Verification items for the finished model (mm, model axes). Give positions to 0.01 mm unless a question says otherwise; leave off trailing zeros. Order: outer loops, then holes, each group sorted by start corner. A loop starts at its lowest first (then second) coordinate and runs counter-clockwise, first axis right, second up. Notation, with made-up numbers: (27, 62.5) -> (48, 62.5) arc R10 cw to (48, 68.5) -> close; hole circle Ø6 at (51.25, 2.5). An arc over 180 degrees is marked (long way). Return JSON: item names as keys, results as strings. Group by question number.
(1) Cross-section at A-A on y = 1.75. Enter the section's corners in (x, z).
(2) Cross-section at B-B on x = 0. State how many separate pieces and enclosed holes the cut face has, then the cut area to 3 significant figures.
(3) Thickness scan on line 1 along Z through (x, y) = (0, 4.45); line 2 along X through (y, z) = (2.25, -70.5); line 3 along X through (y, z) = (-4.15, 265). Record the ranges inside material, lowest first.
(4) Cross-section at C-C on z = 157. Enter the section's corners in (x, y), then the cut area to 3 significant figures.
from build123d import *

# Parameters (mm, degrees)
SKIZZE1_W                       = 10
SKIZZE1_H                       = 10
SKIZZE1_W_2                     = 7
SKIZZE1_H_2                     = 7
AUFSATZ_LINEAR_AUSTRAGEN1_DEPTH = 280
SKIZZE2_R                       = 2.75
SCHNITT_LINEAR_AUSTRAGEN1_DEPTH = 15


with BuildPart() as part:
    # Skizze1 → Aufsatz-Linear austragen1 (new, symmetric)
    with BuildSketch(Plane.XY):
        Rectangle(SKIZZE1_W, SKIZZE1_H)
        Rectangle(SKIZZE1_W_2, SKIZZE1_H_2, mode=Mode.SUBTRACT)
    extrude(amount=AUFSATZ_LINEAR_AUSTRAGEN1_DEPTH, both=True)

    # Skizze2 → Schnitt-Linear austragen1 (cut, symmetric)
    with BuildSketch(Plane(origin=(0, 0, 0), x_dir=(1, 0, 0), z_dir=(0, 1, 0))):
        with Locations((0, -265)):
            Circle(SKIZZE2_R)
        with Locations((0, 265)):
            Circle(SKIZZE2_R)
        with Locations((0, -220)):
            Circle(SKIZZE2_R)
        with Locations((0, 220)):
            Circle(SKIZZE2_R)
    extrude(amount=SCHNITT_LINEAR_AUSTRAGEN1_DEPTH, both=True, mode=Mode.SUBTRACT)


solid = part.part
Verdict:
{
 "1": {"outline": "(-5, -280) -> (-3.5, -280) -> (-3.5, 280) -> (-5, 280) -> close; (3.5, -280) -> (5, -280) -> (5, 280) -> (3.5, 280) -> close"},
 "2": {"separate pieces": "10", "enclosed holes": "0", "area": "1,610 mm²"},
 "3": {"line 1": "-280 to -267.75, -262.25 to -222.75, -217.25 to 217.25, 222.75 to 262.25, 267.75 to 280", "line 2": "-5 to -3.5, 3.5 to 5", "line 3": "-5 to -2.75, 2.75 to 5"},
 "4": {"outline": "(-5, -5) -> (5, -5) -> (5, 5) -> (-5, 5) -> close; hole (-3.5, -3.5) -> (3.5, -3.5) -> (3.5, 3.5) -> (-3.5, 3.5) -> close", "area": "51.0 mm²"}
}
